The drawing under review shows one solid part. Ordinate dimensions are in mm from its lowest x, y, z. Round coordinates to 2 decimals unless told otherwise and drop trailing zeros. Order: outer loops, then holes, each group sorted by start corner. A loop starts at its lowest first (then second) coordinate and runs counter-clockwise, first axis right, second up.
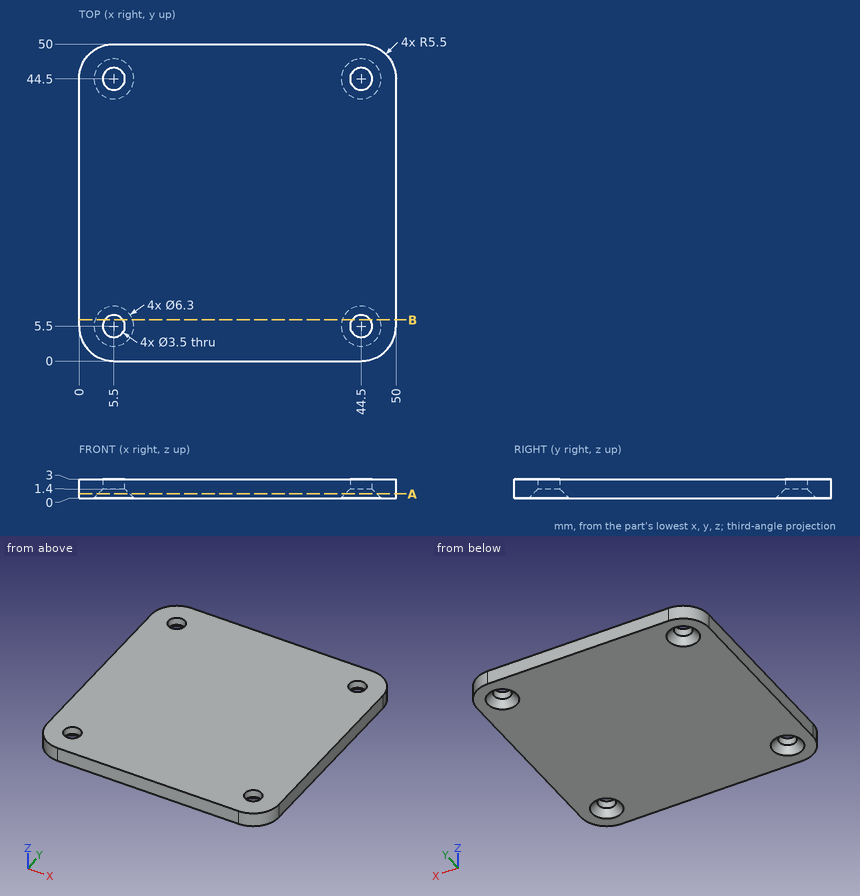
(1) We need section B-B (y = 6.5). Count the separate pieces of the cut face and the enclosed holes in it, and give its area (3 significant figures).
(2) To check wall thickness, follow L1, parallel to Y at x = 44.5, z = 1.85; L2, parallel to Y at x = 4.5, z = 2.7; L3, parallel to X at y = 43, z = 1.1. State the ranges of each line that lie inside material, in increasing order.
(3) Clearance check with flat-ended pins moving along their axes: P1, Ø5.5, axis at x = 5.5, y = 5.5, coming from the -Z side; P2, Ø3, axis at x = 5.5, y = 44.5, coming from the -Z side. State where each tip first meets the part, or that it passes through.
(4) We need section A-A (z = 0.65). Give the boundary of the cut face in (x, y), and give its area (3 significant figures).
Verdict:
1. separate pieces: 3
1. enclosed holes: 0
1. area: 128 mm2
2. L1: y = 0 to 3.75, 7.25 to 42.75, 46.25 to 50
2. L2: y = 0.09 to 4.06, 6.94 to 43.06, 45.94 to 49.91
2. L3: x = 0 to 4.1, 6.9 to 43.1, 45.9 to 50
3. P1: stops at z = 0.4
3. P2: passes through
4. outline: (0, 5.5) arc R5.5 ccw to (5.5, 0) - (44.5, 0) arc R5.5 ccw to (50, 5.5) - (50, 44.5) arc R5.5 ccw to (44.5, 50) - (5.5, 50) arc R5.5 ccw to (0, 44.5) - close; hole circle Ø5 at (5.5, 5.5); hole circle Ø5 at (5.5, 44.5); hole circle Ø5 at (44.5, 5.5); hole circle Ø5 at (44.5, 44.5)
4. area: 2,400 mm2
